The listing builds one solid part. Answer for the finished solid, in the listing's coordinates (mm). A direction names the side the tool comes from. Coordinates: 2 decimals unless noted, no trailing zeros. Write each loop counter-clockwise with the first axis right and the second up, starting at its lowest first coordinate (ties: lowest second). Pieces come first, ordered by that corner, then holes.
from build123d import *

# Parameters (mm, degrees)
EXTRUDE_1_DEPTH     = 1.6
SKETCH_2_R          = 5
EXTRUDE_2_DEPTH     = 6
EXTRUDE_START       = -6
SKETCH_3_R          = 4.25
EXTRUDE_3_DEPTH     = 10.2
SKETCH_4_R          = 0.5
CUT_EXTRUDE_1_DEPTH = 2.6
EXTRUDE_START_2     = -1.6
SKETCH_5_W          = 0.976311431
SKETCH_5_H          = 2.037519509
EXTRUDE_4_DEPTH     = 3.3


with BuildPart() as part:
    # 草图1 → 凸台-拉伸1 (new body)
    with BuildSketch(Plane(origin=(0, 0, 0), x_dir=(1, 0, 0), z_dir=(0, 1, 0))):
        with BuildLine():
            ThreePointArc((7.894379623, -1.295673712), (6.748699348, 0.13250325), (7.837436926, 1.604550536))
            ThreePointArc((7.837436926, 1.604550536), (-0.157040889, 7.998458486), (-7.894379623, 1.295673712))
            ThreePointArc((-7.894379623, 1.295673712), (-6.748699348, -0.13250325), (-7.837436926, -1.604550536))
            ThreePointArc((-7.837436926, -1.604550536), (0.157040889, -7.998458486), (7.894379623, -1.295673712))
        make_face()
    extrude(amount=EXTRUDE_1_DEPTH)

    # 草图2 → 凸台-拉伸2 (add)
    with BuildSketch(Plane(origin=(0, 1.6, 0), x_dir=(1, 0, 0), z_dir=(0, 1, 0))):
        Circle(SKETCH_2_R)
    extrude(amount=EXTRUDE_2_DEPTH)

    # 草图3 → 凸台-拉伸3 (add)
    with BuildSketch(Plane(origin=(0, 7.6, 0), x_dir=(1, 0, 0), z_dir=(0, 1, 0)).offset(EXTRUDE_START)):
        Circle(SKETCH_3_R)
    extrude(amount=EXTRUDE_3_DEPTH)

    # 草图4 → 切除-拉伸1 (cut, through all)
    with BuildSketch(Plane(origin=(0, 1.6, 0), x_dir=(1, 0, 0), z_dir=(0, 1, 0))):
        with Locations((-2.54, 6.380087041)):
            Circle(SKETCH_4_R)
        with Locations((0, 6.380087041)):
            Circle(SKETCH_4_R)
        with Locations((2.54, 6.380087041)):
            Circle(SKETCH_4_R)
    extrude(amount=-CUT_EXTRUDE_1_DEPTH, mode=Mode.SUBTRACT)

    # 草图5 → 凸台-拉伸4 (add)
    with BuildSketch(Plane.XZ.offset(EXTRUDE_START_2)):
        with Locations((5.05135045, -3.862797403)):
            Rectangle(SKETCH_5_W, SKETCH_5_H)
    extrude(amount=EXTRUDE_4_DEPTH)


solid = part.part
Q1. The part is cut by section A-A, the plane x = 0. Write down the section's boundary in (y, z), then the cut area to 3 significant figures.
Answers below:
outline: (0, -8) - (1.6, -8) - (1.6, -6.88) - (0, -6.88) - close; (0, -5.88) - (1.6, -5.88) - (1.6, -5) - (7.6, -5) - (7.6, -4.25) - (11.8, -4.25) - (11.8, 4.25) - (7.6, 4.25) - (7.6, 5) - (1.6, 5) - (1.6, 8) - (0, 8) - close
area: 120 mm2
Q2. Which of the six approach directions +Z, -Z, +X, -X, +Y, -Y give full straight-line access (tool end or side, diameter ignored) to faces 1 (the face through (4.563, -1, -4)), 2 (the face through (5.54, -1, -4)), 3 (the face through (-1.08, 4.56, 4.88)), 4 (the face through (5, -1, -2.844))?
Answers below:
face 1: +Z, -Z, -X, -Y
face 2: +Z, -Z, +X, -Y
face 3: +Y
face 4: +Z, +X, -X, -Y
Q3. The part is cut by section D-D, the plane z = 0. Write down the section's boundary in (x, y), then the cut area to 3 significant figures.
Answers below:
outline: (-6.76, 0) - (6.76, 0) - (6.76, 1.6) - (5, 1.6) - (5, 7.6) - (4.25, 7.6) - (4.25, 11.8) - (-4.25, 11.8) - (-4.25, 7.6) - (-5, 7.6) - (-5, 1.6) - (-6.76, 1.6) - close
area: 117 mm2
Q4. Given pin 1 (8 mm diameter, centred on y = 9.5, z = 4, fed in from +X); pin 2 (3 mm diameter, centred on x = 0.5, y = 7, fed in from +Z); pin 3 (3 mm diameter, centred on x = 5.5, y = 7, fed in from -Z), each flat-ended and moving along its own axis, determine where each tip first touches the part or whether it passes through.
Answers below:
pin 1: stops at x = 4.98
pin 2: stops at z = 5
pin 3: stops at z = -3
Q5. Find the intervals of material crossed by probe 1 along Z at (x, y) = (0, 0.7); probe 2 along Y at (x, z) = (2.5, -3.25); probe 3 along Z at (x, y) = (2.54, 0.95), in increasing order.
Answers below:
probe 1: z = -8 to -6.88, -5.88 to 8
probe 2: y = 0 to 11.8
probe 3: z = -7.59 to -6.88, -5.88 to 7.59
Q6. The part is cut by section B-B, the plane y = 0.5. Write down the section's boundary in (x, z).
Answers below:
outline: (-7.89, -1.3) arc R8 ccw to (7.84, -1.6) arc R1.5 cw to (7.89, 1.3) arc R8 ccw to (-7.84, 1.6) arc R1.5 cw to start; hole circle Ø1 at (-2.54, -6.38); hole circle Ø1 at (0, -6.38); hole circle Ø1 at (2.54, -6.38)
Q7. The part is cut by section C-C, the plane x = -2.5. Write down the section's boundary in (y, z), then the cut area to 3 significant figures.
Answers below:
outline: (0, -7.6) - (1.6, -7.6) - (1.6, -6.88) - (0, -6.88) - close; (0, -5.88) - (1.6, -5.88) - (1.6, -4.33) - (7.6, -4.33) - (7.6, -3.44) - (11.8, -3.44) - (11.8, 3.44) - (7.6, 3.44) - (7.6, 4.33) - (1.6, 4.33) - (1.6, 7.6) - (0, 7.6) - close
area: 104 mm2
